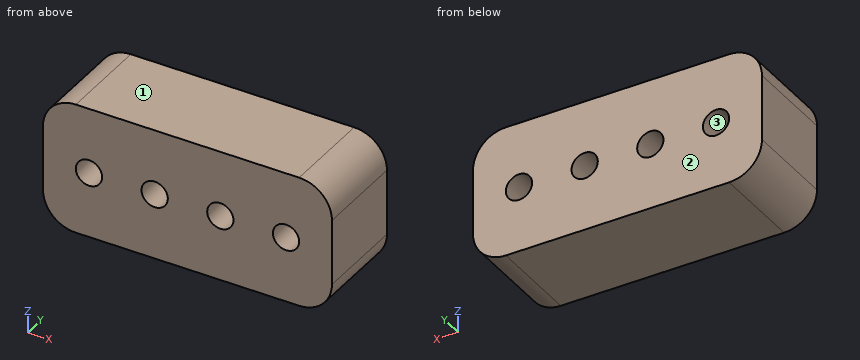
Autodesk Inventor part; units mm, degrees
ref_plane "YZ Plane" through (0, 0, 0) normal (1, 0, 0) x (0, 1, 0)
ref_plane "XZ Plane" through (0, 0, 0) normal (0, 1, 0) x (-1, 0, 0)
ref_plane "XY Plane" through (0, 0, 0) normal (0, 0, 1) x (1, 0, 0)
sketch "Sketch1" plane through (0, 0, 0) normal (0, 1, 0) x (-1, 0, 0)
  line L0 (6.35, 0) -> (49.53, 0)
  line L1 (55.88, -6.35) -> (55.88, -19.05)
  line L2 (49.53, -25.4) -> (6.35, -25.4)
  line L3 (0, -19.05) -> (0, -6.35)
  circle A0 centre (46.99, -12.7) radius 2.54
  circle A1 centre (34.29, -12.7) radius 2.54
  circle A2 centre (21.59, -12.7) radius 2.54
  circle A3 centre (8.89, -12.7) radius 2.54
  line L4 (46.99, -12.7) -> (8.89, -12.7) construction
  arc A4 (49.53, -25.4) -> (55.88, -19.05) centre (49.53, -19.05) ccw
  arc A5 (55.88, -6.35) -> (49.53, 0) centre (49.53, -6.35) ccw
  arc A6 (6.35, 0) -> (0, -6.35) centre (6.35, -6.35) ccw
  arc A7 (0, -19.05) -> (6.35, -25.4) centre (6.35, -19.05) ccw
  point P0 (0, 0)
  dimension "d0" = 25.4
  dimension "d1" = 55.88
  dimension "d2" = 5.08
  dimension "d3" = 12.7
  dimension "d4" = 12.7
  dimension "d5" = 12.7
  dimension "d6" = 12.7
  dimension "d7" = 8.89
  dimension "d8" = 6.35
extrude "Extrusion1" add sketch "Sketch1" along normal blind 17.78
properties part number "ELEV_023_BILLET2" material "Aluminum 6061"
Here's how the part is built. I have some questions about the finished solid (model axes, mm). Face numbers are marked on the shaded views. Give positions to 0.01 mm unless a question says otherwise; leave off trailing zeros. Order: outer loops, then holes, each group sorted by start corner. A loop starts at its lowest first (then second) coordinate and runs counter-clockwise, first axis right, second up. Notation, with made-up numbers: M 45.5,29 L 101.5,29 A26 cw 101.5,68 Z; hole C -9.5,67 d10. An arc over 180 degrees is marked long. Use a Markdown table: item, result. Add a question column.
1. I need wall thicknesses on probe 1 along Z at (x, y) = (-46.99, 9.75); probe 2 along X at (y, z) = (7.5, -13.25); probe 3 along Z at (x, y) = (-46, 1.5). Which ranges of each line are inside material? Lowest first, please. Write a range as from..to.
2. Suppose I cut it at B-B (z = -12.7). List the corners of the cut face in (x, y) for me, and give its area (3 significant figures).
3. For pin 1 Ø3 at (x, z) = (-21.59, -12.7) entering from +Y, with a flat end and sliding along its axis, tell me the tip position at first contact or that it passes through.
4. Suppose I cut it at D-D (x = -23). List the corners of the cut face in (y, z) for me.
5. If we mould it in two halves opening along Z, with no side actions, what happens to the marked faces 1, 2 and 3? For each: +Z half, -Z half, draft (parallel to the pull), parting line (faces both ways), or undercut.
6. Suppose I cut it at C-C (y = 16.5). List the corners of the cut face in (x, z) for me, and give its area (3 significant figures).
7. Suppose I cut it at A-A (x = -46.99). List the corners of the cut face in (y, z) for me.
Results list:
| question | item | result |
|---|---|---|
| 1 | probe 1 | z = -25.4..-15.24, -10.16..0 |
| 1 | probe 2 | x = -55.88..-49.47, -44.51..-36.77, -31.81..-24.07, -19.11..-11.37, -6.41..0 |
| 1 | probe 3 | z = -25.4..-15.04, -10.36..0 |
| 2 | outline | M -55.88,0 L -49.53,0 L -49.53,17.78 L -55.88,17.78 Z; M -44.45,0 L -36.83,0 L -36.83,17.78 L -44.45,17.78 Z; M -31.75,0 L -24.13,0 L -24.13,17.78 L -31.75,17.78 Z; M -19.05,0 L -11.43,0 L -11.43,17.78 L -19.05,17.78 Z; M -6.35,0 L 0,0 L 0,17.78 L -6.35,17.78 Z |
| 2 | area | 632 mm² |
| 3 | pin 1 | passes through |
| 4 | outline | M 0,-25.4 L 17.78,-25.4 L 17.78,-14.81 L 0,-14.81 Z; M 0,-10.59 L 17.78,-10.59 L 17.78,0 L 0,0 Z |
| 5 | face 1 | +Z half |
| 5 | face 2 | draft |
| 5 | face 3 | undercut |
| 6 | outline | M -55.88,-19.05 A6.35 ccw -49.53,-25.4 L -6.35,-25.4 A6.35 ccw 0,-19.05 L 0,-6.35 A6.35 ccw -6.35,0 L -49.53,0 A6.35 ccw -55.88,-6.35 Z; hole C -46.99,-12.7 d5.08; hole C -34.29,-12.7 d5.08; hole C -21.59,-12.7 d5.08; hole C -8.89,-12.7 d5.08 |
| 6 | area | 1,300 mm² |
| 7 | outline | M 0,-25.4 L 17.78,-25.4 L 17.78,-15.24 L 0,-15.24 Z; M 0,-10.16 L 17.78,-10.16 L 17.78,0 L 0,0 Z |
